Geometry: see drawing. Coordinates: mm, zero at the bounding-box minimum. Give positions to 0.01 mm unless a question says otherwise; leave off trailing zeros. Loops run counter-clockwise (first coordinate to the right, second up) from the corner with the lowest first, then second, coordinate; pieces in that order, holes last. Notation, with made-up numbers: M 23.5,-0.75 L 61.5,-0.75 A30 cw 61.5,29.25 Z; hole C -30.5,-29.75 d9. An arc over 180 degrees is marked long. Put each result on its own line as item: value.
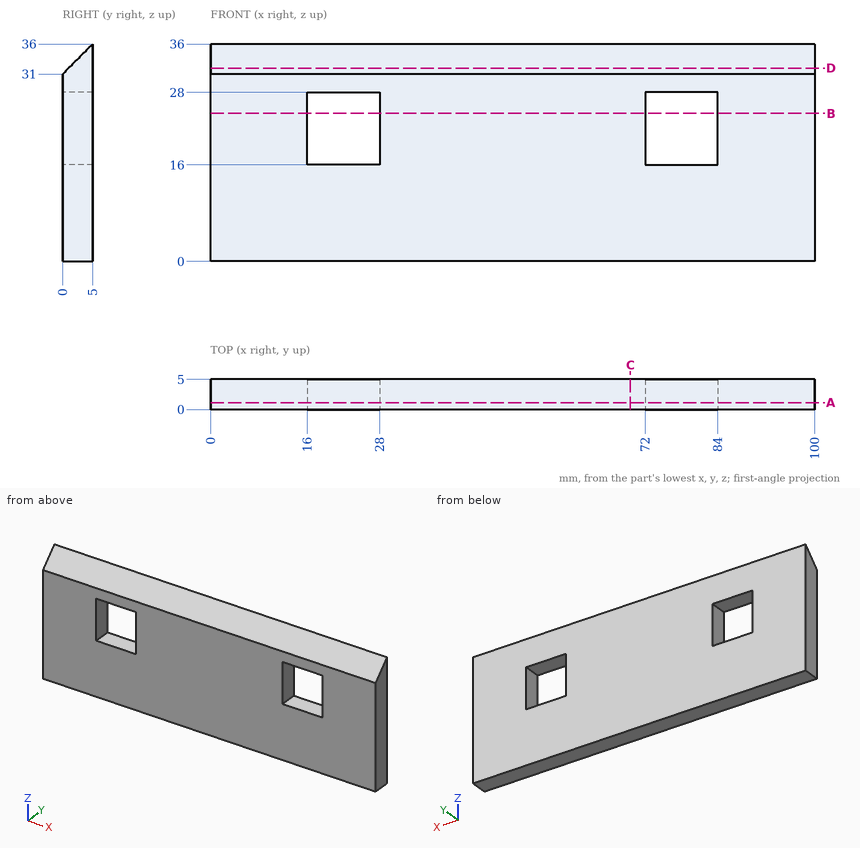
1. Section query A-A (y = 1.15). Output: boundary loops of the cut face in (x, z).
Found:
outline: M 0,0 L 100,0 L 100,32.15 L 0,32.15 Z; hole M 16,16 L 28,16 L 28,28 L 16,28 Z; hole M 72,16 L 84,16 L 84,28 L 72,28 Z
2. Contact query for a flat-ended pin moving along its axis: P1, Ø1.5, axis at x = 20.5, y = 2.5, coming from the +Z side. Output: stop coordinate, or through.
Found:
P1: z = 34.25
3. Material intervals for line 1 (X direction, y = 1.85, z = 21); line 2 (Z direction, x = 24.5, y = 0.5); line 3 (Z direction, x = 56, y = 1.9), sorted ascending. Write a range as from..to.
Found:
line 1: 0..16, 28..72, 84..100
line 2: 0..16, 28..31.5
line 3: 0..32.9
4. Section query C-C (x = 69.5). Output: boundary loops of the cut face in (y, z).
Found:
outline: M 0,0 L 5,0 L 5,36 L 0,31 Z
5. Section query D-D (z = 32). Output: boundary loops of the cut face in (x, y).
Found:
outline: M 0,1 L 100,1 L 100,5 L 0,5 Z
6. Section query B-B (z = 24.5). Output: boundary loops of the cut face in (x, y), plus the area to 3 significant figures.
Found:
outline: M 0,0 L 16,0 L 16,5 L 0,5 Z; M 28,0 L 72,0 L 72,5 L 28,5 Z; M 84,0 L 100,0 L 100,5 L 84,5 Z
area: 380 mm^2
